Here's how the part is built. I have some questions about the finished solid (model axes, mm). Round coordinates to 2 decimals unless told otherwise and drop trailing zeros. Write each loop counter-clockwise with the first axis right and the second up, starting at its lowest first coordinate (ties: lowest second). Pieces come first, ordered by that corner, then holes. Notation, with made-up numbers: (26.5, 82.5) - (84.5, 82.5) arc R31 cw to (84.5, 109.5) - close; hole circle Ø2 at (4, 63.25). An arc over 180 degrees is marked (long way). One line per item, written item: value. Start each with the question number.
Item 1: Imagine slicing it at C-C, the plane y = -26. Please give me the cut outline in (x, z).
Item 2: Imagine slicing it at A-A, the plane y = 0. Please give me the cut outline in (x, z), then the cut area to 3 significant figures.
Item 3: If I drill on line 1 (Y direction, x = -5.5, z = -0.7); line 2 (X direction, y = 0, z = -1.25); line 3 (X direction, y = 27, z = -0.25), over which ranges is the centre line in solid material (lowest first)?
Item 4: Imagine slicing it at B-B, the plane x = -13.5. Please give me the cut outline in (y, z), then the cut area to 3 significant figures.
Item 5: For P1, Ø1, axis at x = 36, z = -1, coming from the -Y side; P2, Ø0.6, axis at y = 34.5, z = -1.5, coming from the -X side; P3, Ø1.5, axis at x = -22, y = 8.5, coming from the +Z side; P4, Ø1, axis at x = 36, z = -1.5, coming from the +Y side, each with a flat end and sliding along its axis, tell me the tip position at first contact or that it passes through.
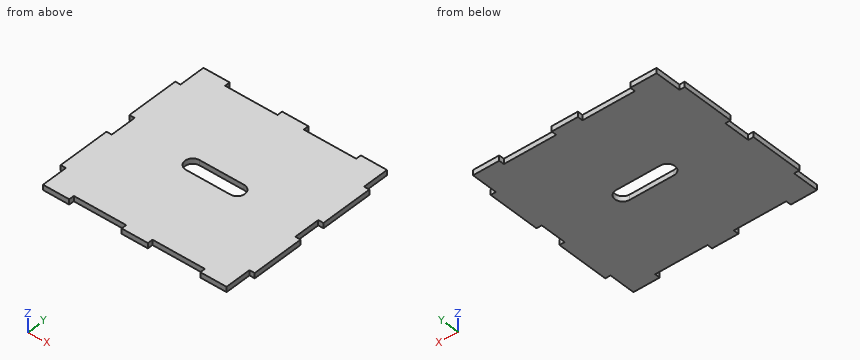
```python
from build123d import *

# Parameters (mm, degrees)
SKETCH1_W           = 70
SKETCH1_H           = 70
BOSS_EXTRUDE1_DEPTH = 2
SKETCH2_W           = 2
SKETCH2_H           = 20
BOSS_EXTRUDE2_DEPTH = 2
SKETCH3_W           = 20
SKETCH3_H           = 2
CUT_EXTRUDE1_DEPTH  = 2
SKETCH4_W           = 16.92
SKETCH4_H           = 5.9
CUT_EXTRUDE2_DEPTH  = 10


with BuildPart() as part:
    # Sketch1 → Boss-Extrude1 (new body)
    with BuildSketch(Plane.XY):
        Rectangle(SKETCH1_W, SKETCH1_H)
    extrude(amount=-BOSS_EXTRUDE1_DEPTH)

    # Sketch2 → Boss-Extrude2 (add)
    with BuildSketch(Plane.XY):
        with Locations((-36, 15)):
            Rectangle(SKETCH2_W, SKETCH2_H)
        with Locations((-36, -15)):
            Rectangle(SKETCH2_W, SKETCH2_H)
        with Locations((36, -15)):
            Rectangle(SKETCH2_W, SKETCH2_H)
        with Locations((36, 15)):
            Rectangle(SKETCH2_W, SKETCH2_H)
    extrude(amount=-BOSS_EXTRUDE2_DEPTH)

    # Sketch3 → Cut-Extrude1 (cut)
    with BuildSketch(Plane.XY):
        with Locations((-15, 34)):
            Rectangle(SKETCH3_W, SKETCH3_H)
        with Locations((15, 34)):
            Rectangle(SKETCH3_W, SKETCH3_H)
        with Locations((-15, -34)):
            Rectangle(SKETCH3_W, SKETCH3_H)
        with Locations((15, -34)):
            Rectangle(SKETCH3_W, SKETCH3_H)
    extrude(amount=-CUT_EXTRUDE1_DEPTH, mode=Mode.SUBTRACT)

    # Sketch4 → Cut-Extrude2 (cut)
    with BuildSketch(Plane.XY):
        Rectangle(SKETCH4_W, SKETCH4_H)
        with BuildLine():
            ThreePointArc((8.46, 2.95), (11.41, 0), (8.46, -2.95))
            Line((8.46, -2.95), (8.46, 2.95))
        make_face()
        with BuildLine():
            Line((-8.46, -2.95), (-8.46, 2.95))
            ThreePointArc((-8.46, 2.95), (-11.41, 0), (-8.46, -2.95))
        make_face()
    extrude(amount=-CUT_EXTRUDE2_DEPTH, mode=Mode.SUBTRACT)


solid = part.part
```
Values follow:
1. outline: (-35, -2) - (35, -2) - (35, 0) - (-35, 0) - close
2. outline: (-35, -2) - (-11.41, -2) - (-11.41, 0) - (-35, 0) - close; (11.41, -2) - (35, -2) - (35, 0) - (11.41, 0) - close
2. area: 94.4 mm^2
3. line 1: y = -33 to -2.95, 2.95 to 33
3. line 2: x = -35 to -11.41, 11.41 to 35
3. line 3: x = -35 to 35
4. outline: (-33, -2) - (33, -2) - (33, 0) - (-33, 0) - close
4. area: 132 mm^2
5. P1: stops at y = -25
5. P2: stops at x = -35
5. P3: stops at z = 0
5. P4: stops at y = 25
